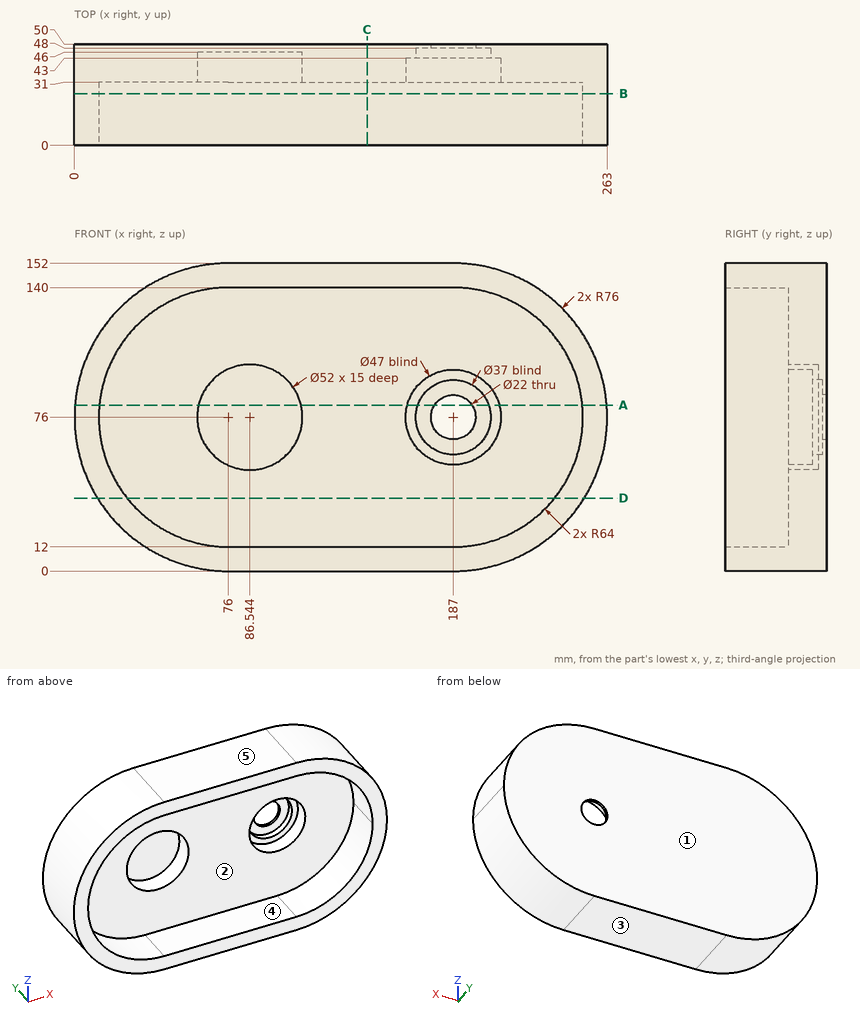
Source: three-view drawing plus pictorial views. Frame: mm from the lowest corner of the part. A direction names the side the tool comes from. Round coordinates to 2 decimals unless told otherwise and drop trailing zeros. Loops run counter-clockwise (first coordinate to the right, second up) from the corner with the lowest first, then second, coordinate; pieces in that order, holes last. Notation, with made-up numbers: M 22.25,76.5 L 59.25,76.5 A17 cw 59.25,106.5 Z; hole C 70,6 d10. An arc over 180 degrees is marked long. Put each result on its own line as item: value. Start each with the question number.
(1) Draft query along Z for the marked faces 3, 4 and 5. Return one class per face: +Z half, -Z half, draft (parallel to the pull), parting line (faces both ways), or undercut.
(2) Set-up query: the marked faces 1 and 2. Return all of +Z, -Z, +X, -X, +Y, -Y with unobstructed straight access to the full face (end or side cutting, diameter ignored); none if empty.
(3) Section query A-A (z = 82). Return loops of the section in (x, y), then the cut area to 3 significant figures.
(4) Section query B-B (y = 25.5). Return loops of the section in (x, z).
(5) Material intervals for line 1 along Z through (x, y) = (117.5, 22); line 2 along X through (y, z) = (48.95, 76); line 3 along Y through (x, z) = (235, 36.5), sorted ascending. Write a range as [from, to].
(6) Section query C-C (x = 144.5). Return loops of the section in (y, z), then the cut area to 3 significant figures.
(7) Contact query for flat-ended pins moving along their axis: pin 1 Ø1.5 at (x, z) = (143.5, 52.5) entering from -Y; pin 2 Ø3 at (y, z) = (13, 16) entering from +X (1 decimal); pin 3 Ø3 at (y, z) = (36, 82) entering from -X. Output: stop coordinate, or through.
(8) Section query D-D (z = 36). Return loops of the section in (x, y).
Findings below:
1. face 3: -Z half
1. face 4: undercut
1. face 5: +Z half
2. face 1: +Z, -Z, +X, -X, +Y
2. face 2: -Y
3. outline: M 0.24,0 L 12.28,0 L 12.28,31 L 61.25,31 L 61.25,46 L 111.84,46 L 111.84,31 L 164.28,31 L 164.28,43 L 169.5,43 L 169.5,48 L 177.78,48 L 177.78,50 L 0.24,50 Z; M 196.22,48 L 204.5,48 L 204.5,43 L 209.72,43 L 209.72,31 L 250.72,31 L 250.72,0 L 262.76,0 L 262.76,50 L 196.22,50 Z
3. area: 4,220 mm2
4. outline: M 76,0 L 187,0 A76 ccw 187,152 L 76,152 A76 ccw Z; hole M 76,12 L 187,12 A64 ccw 187,140 L 76,140 A64 ccw Z
5. line 1: z = [0, 12], [140, 152]
5. line 2: x = [0, 176], [198, 263]
5. line 3: y = [31, 50]
6. outline: M 0,0 L 50,0 L 50,152 L 0,152 L 0,140 L 31,140 L 31,12 L 0,12 Z
6. area: 3,630 mm2
7. pin 1: stops at y = 31
7. pin 2: stops at x = 235.5
7. pin 3: stops at x = 0.13
8. outline: M 11.38,0 L 26.04,0 L 26.04,31 L 236.96,31 L 236.96,0 L 251.62,0 L 251.62,50 L 11.38,50 Z
